```python
from build123d import *

# Parameters (mm, degrees)
SKETCH1_W           = 80
SKETCH1_H           = 90
BOSS_EXTRUDE1_DEPTH = 3.175
SKETCH2_W           = 5
SKETCH2_H           = 3.175
BOSS_EXTRUDE2_DEPTH = 2.5
SKETCH3_W           = 3.175
SKETCH3_H           = 5
BOSS_EXTRUDE3_DEPTH = 2.5
SKETCH4_W           = 3.175
SKETCH4_H           = 5
BOSS_EXTRUDE4_DEPTH = 2.5
LPATTERN1_COUNT     = 9
LPATTERN1_PITCH     = 10
LPATTERN2_COUNT     = 8
LPATTERN2_PITCH     = 10
LPATTERN3_COUNT     = 9
LPATTERN3_PITCH     = 10


with BuildPart() as part:
    # Sketch1 → Boss-Extrude1 (new body)
    with BuildSketch(Plane.XY):
        with Locations((40, 45)):
            Rectangle(SKETCH1_W, SKETCH1_H)
    extrude(amount=BOSS_EXTRUDE1_DEPTH)

    # Sketch2 → Boss-Extrude2 (add)
    with BuildSketch(Plane.XZ):
        with Locations((2.5, 1.5875)):
            Rectangle(SKETCH2_W, SKETCH2_H)
    boss_extrude2 = extrude(amount=BOSS_EXTRUDE2_DEPTH)

    # Sketch3 → Boss-Extrude3 (add)
    with BuildSketch(Plane(origin=(80, 0, 0), x_dir=(0, 0, -1), z_dir=(1, 0, 0))):
        with Locations((-1.5875, 87.5)):
            Rectangle(SKETCH3_W, SKETCH3_H)
    boss_extrude3 = extrude(amount=BOSS_EXTRUDE3_DEPTH)

    # Sketch4 → Boss-Extrude4 (add)
    with BuildSketch(Plane.ZY):
        with Locations((1.5875, 87.5)):
            Rectangle(SKETCH4_W, SKETCH4_H)
    boss_extrude4 = extrude(amount=BOSS_EXTRUDE4_DEPTH)

    # LPattern1: Boss-Extrude4 ×9
    with Locations(*[(0, -i * LPATTERN1_PITCH, 0) for i in range(1, LPATTERN1_COUNT)]):
        add(boss_extrude4)

    # LPattern2: Boss-Extrude2 ×8
    with Locations(*[(i * LPATTERN2_PITCH, 0, 0) for i in range(1, LPATTERN2_COUNT)]):
        add(boss_extrude2)

    # LPattern3: Boss-Extrude3 ×9
    with Locations(*[(0, -i * LPATTERN3_PITCH, 0) for i in range(1, LPATTERN3_COUNT)]):
        add(boss_extrude3)


solid = part.part
```
Input: part model. Units: mm. Frame: model coordinates. A direction names the side the tool comes from. Coordinates: 2 decimals unless noted, no trailing zeros. Order: outer loops, then holes, each group sorted by start corner. A loop starts at its lowest first (then second) coordinate and runs counter-clockwise, first axis right, second up. Notation, with made-up numbers: (-5.5, 19) - (27.5, 19) arc R14 cw to (27.5, 24) - close; hole circle Ø1 at (-17.5, 61). An arc over 180 degrees is marked (long way). Return JSON: item names as keys, results as strings.
Q1. Ray query, probe 1 along Y at (x, z) = (17, 2.85); probe 2 along X at (y, z) = (3.5, 2.1). Return the intervals inside material, ascending.
The answers:
{"probe 1": "y = 0 to 90", "probe 2": "x = 0 to 80"}
Q2. First-contact query: pin 1 (1.6 mm diameter, centred on x = 18, z = 2, fed in from -Y); pin 2 (1.6 mm diameter, centred on y = 3, z = 2, fed in from +X); pin 3 (0.8 mm diameter, centred on x = 81, z = 1, fed in from -Y). Flat tips, straight axial feed; report the tip coordinate or a pass-through.
The answers:
{"pin 1": "stops at y = 0", "pin 2": "stops at x = 80", "pin 3": "stops at y = 5"}
Q3. Cut plane A-A (x = 7.5). Return loops of the section in (y, z) (3 decimals).
The answers:
{"outline": "(0, 0) - (90, 0) - (90, 3.175) - (0, 3.175) - close"}
Q4. Draft query along Y for faces 5 (the flat face through (42, -2.5, 2)), 6 (the flat face through (82.5, 68, 2)), 7 (the flat face through (-1, 30, 2)). Return one class per face: +Y half, -Y half, draft (parallel to the pull), parting line (faces both ways), or undercut.
The answers:
{"face 5": "-Y half", "face 6": "draft", "face 7": "undercut"}
Q5. Cut plane B-B (y = 22). Return loops of the section in (x, z) (3 decimals), then the cut area to 3 significant figures.
The answers:
{"outline": "(0, 0) - (80, 0) - (80, 3.175) - (0, 3.175) - close", "area": "254 mm2"}
Q6. Access query for faces 1 (the flat face through (60, -1, 2)), 2 (the flat face through (-1, 45, 2)), 3 (the flat face through (81, 50, 2)), 4 (the flat face through (-1, 5, 2)). Directions: +Z, -Z, +X, -X, +Y, -Y. A direction counts if a zero-diameter tool reaches every point of the face in a straight line with its end or side. Return the directions, or none.
The answers:
{"face 1": "+Z, -Z, -Y", "face 2": "+Z, -Z, -X", "face 3": "+Z, -Z, +X", "face 4": "+Z, -Z, -X, -Y"}
